from build123d import *

# Parameters (mm, degrees)
SKETCH1_W           = 239.014
SKETCH1_H           = 177.8
BOSS_EXTRUDE1_DEPTH = 127
SKETCH2_W           = 232.664
SKETCH2_H           = 171.45
CUT_EXTRUDE1_DEPTH  = 123.825
SKETCH3_W           = 177.8
SKETCH3_H           = 6.35
BOSS_EXTRUDE2_DEPTH = 38.1
SKETCH5_R           = 3.175
CUT_EXTRUDE2_DEPTH  = 6.35


with BuildPart() as part:
    # Sketch1 → Boss-Extrude1 (new body)
    with BuildSketch(Plane(origin=(0, 0, 0), x_dir=(1, 0, 0), z_dir=(0, 1, 0))):
        Rectangle(SKETCH1_W, SKETCH1_H)
    extrude(amount=BOSS_EXTRUDE1_DEPTH)

    # Sketch2 → Cut-Extrude1 (cut)
    with BuildSketch(Plane(origin=(0, 127, 0), x_dir=(1, 0, 0), z_dir=(0, 1, 0))):
        Rectangle(SKETCH2_W, SKETCH2_H)
    extrude(amount=-CUT_EXTRUDE1_DEPTH, mode=Mode.SUBTRACT)

    # Sketch3 → Boss-Extrude2 (add)
    with BuildSketch(Plane(origin=(119.507, 0, 0), x_dir=(0, 0, -1), z_dir=(1, 0, 0))):
        with Locations((0, 123.825)):
            Rectangle(SKETCH3_W, SKETCH3_H)
    extrude(amount=BOSS_EXTRUDE2_DEPTH)

    # Sketch5 → Cut-Extrude2 (cut)
    with BuildSketch(Plane(origin=(0, 127, 0), x_dir=(1, 0, 0), z_dir=(0, 1, 0))):
        with Locations(Location((136.9695, 0, 0), (0, 0, 270))):
            Circle(SKETCH5_R)
    extrude(amount=-CUT_EXTRUDE2_DEPTH, mode=Mode.SUBTRACT)


solid = part.part
For this review, take the finished solid that the model builds, in its own axes (mm). A direction names the side the tool comes from. Round coordinates to 2 decimals unless told otherwise and drop trailing zeros. Order: outer loops, then holes, each group sorted by start corner. A loop starts at its lowest first (then second) coordinate and runs counter-clockwise, first axis right, second up. Notation, with made-up numbers: (82, -25) -> (89, -25) arc R28 ccw to (89, 5) -> close; hole circle Ø3 at (-13.75, 88). An arc over 180 degrees is marked (long way). Write item = value, one per line. Start each with the question number.
1) To check wall thickness, follow line 1 (X direction, y = 125, z = 0); line 2 (Z direction, x = 44.5, y = 24) (3 decimals); line 3 (X direction, y = 10, z = 4). State the ranges of each line that lie inside material, in increasing order. Write a range as from..to.
2) Tool access review of faces 5 (the face through (-2, 66, 85.725)), 6 (the face through (121, 127, 14)): name each direction out of +Z, -Z, +X, -X, +Y, -Y from which nothing blocks a thin tool from reaching the whole face with its end or side.
3) The part is to be moulded in two halves that separate along X. For faces 1 (the face through (143, 120.65, 1)), 2 (the face through (119.507, 59, 1)), 3 (the face through (-2, 66, -85.725)), 4 (the face through (-119.507, 63, 1)), say which applies: +X half, -X half, draft (parallel to the pull), parting line (faces both ways), or undercut.
4) Take a section at C-C on x = 30. State the section outline as (y, z) points (3 decimals).
5) Take a section at B-B on y = 95.5. State the section outline as (x, z) points (3 decimals), plus the area to 3 significant figures.
6) Insertion check: pin 1 (12 mm diameter, centred on y = 92, z = 26, fed in from +X); pin 2 (11.5 mm diameter, centred on x = 144.5, z = -11, fed in from -Y); pin 3 (10 mm diameter, centred on x = 65.5, z = 9, fed in from +Y) (3 decimals). Each pin has a flat end and moves straight along its axis. Give the tip position at first contact, or say it passes through.
7) Take a section at D-D on z = 62. State the section outline as (x, y) points (3 decimals), plus the area to 3 significant figures.
Verdict:
q1.line_1 = -119.51..-116.33, 116.33..133.79, 140.14..157.61
q1.line_2 = -88.9..-85.725, 85.725..88.9
q1.line_3 = -119.51..-116.33, 116.33..119.51
q2.face_5 = +Y
q2.face_6 = +Z, -Z, +X, -X, +Y
q3.face_1 = draft
q3.face_2 = +X half
q3.face_3 = undercut
q3.face_4 = -X half
q4.outline = (0, -88.9) -> (127, -88.9) -> (127, -85.725) -> (3.175, -85.725) -> (3.175, 85.725) -> (127, 85.725) -> (127, 88.9) -> (0, 88.9) -> close
q5.outline = (-119.507, -88.9) -> (119.507, -88.9) -> (119.507, 88.9) -> (-119.507, 88.9) -> close; hole (-116.332, -85.725) -> (116.332, -85.725) -> (116.332, 85.725) -> (-116.332, 85.725) -> close
q5.area = 2,610 mm2
q6.pin_1 = 119.51
q6.pin_2 = 120.65
q6.pin_3 = 3.175
q7.outline = (-119.507, 0) -> (119.507, 0) -> (119.507, 120.65) -> (157.607, 120.65) -> (157.607, 127) -> (116.332, 127) -> (116.332, 3.175) -> (-116.332, 3.175) -> (-116.332, 127) -> (-119.507, 127) -> close
q7.area = 1,790 mm2
